CAD build for the part. Positions are in the model's coordinates, mm. Face numbers are marked on the shaded views. Round coordinates to 2 decimals unless told otherwise and drop trailing zeros. Loops run counter-clockwise (first coordinate to the right, second up) from the corner with the lowest first, then second, coordinate; pieces in that order, holes last. Notation, with made-up numbers: M 11.5,-25 L 27.5,-25 A19 cw 27.5,-17 Z; hole C -24,-36 d6. An arc over 180 degrees is marked long. Put each result on its own line as item: value. Start each with the question number.
from build123d import *
from build123d.topology import SkipClean

# Parameters (mm, degrees)
SCHIZZO1_R                   = 135
ESTRUSIONE_ESTRUSIONE2_DEPTH = 3
SCHIZZO4_R                   = 132
TAGLIO_ESTRUSIONE1_DEPTH     = 191.942399692
ESTRUSIONE_ESTRUSIONE3_DEPTH = 8
RIPETIZIONECIRCOLARE2_COUNT  = 4
ESTRUSIONE_ESTRUSIONE5_START = -3
ESTRUSIONE_ESTRUSIONE5_DEPTH = 3
RIPETIZIONECIRCOLARE4_COUNT  = 4
ESTRUSIONE_ESTRUSIONE6_START = 5
SCHIZZO9_R                   = 135
ESTRUSIONE_ESTRUSIONE6_DEPTH = 5
SCHIZZO10_R                  = 62.5
TAGLIO_ESTRUSIONE2_DEPTH     = 10
SCHIZZO11_R                  = 2.05
TAGLIO_ESTRUSIONE3_DEPTH     = 10


with BuildPart() as part:
    # Schizzo1 → Estrusione-Estrusione2 (new body)
    with BuildSketch(Plane.XY):
        Circle(SCHIZZO1_R)
    extrude(amount=ESTRUSIONE_ESTRUSIONE2_DEPTH)

    # Schizzo4 → Taglio-Estrusione1 (cut, through all)
    with BuildSketch(Plane.XY.offset(3)):
        Circle(SCHIZZO4_R)
    extrude(amount=-TAGLIO_ESTRUSIONE1_DEPTH, mode=Mode.SUBTRACT)

    # Schizzo5 → Estrusione-Estrusione3 (add)
    with SkipClean():  # the faces are left unmerged after this step: merging them gives an invalid solid
        with BuildSketch(Plane(origin=(0, 0, 0), x_dir=(-1, 0, 0), z_dir=(0, 0, -1))):
            with BuildLine():
                Line((-12.5, 134.420050588), (-12.5, 122.5))
                Line((-12.5, 122.5), (12.5, 122.5))
                Line((12.5, 122.5), (12.5, 134.420050588))
                ThreePointArc((12.5, 134.420050588), (0, 135), (-12.5, 134.420050588))
            make_face()
        estrusione_estrusione3 = extrude(amount=-ESTRUSIONE_ESTRUSIONE3_DEPTH)

    # RipetizioneCircolare2: Estrusione-Estrusione3 ×4 about axis
    with SkipClean():  # the faces are left unmerged after this step: merging them gives an invalid solid
        ripetizionecircolare2_axis = Axis((0, 0, 0), (0, 0, 1))
        for i in range(1, RIPETIZIONECIRCOLARE2_COUNT):
            add(estrusione_estrusione3.rotate(ripetizionecircolare2_axis, i * 360 / RIPETIZIONECIRCOLARE2_COUNT))

    # Schizzo8 → Estrusione-Estrusione5 (add)
    with SkipClean():  # the faces are left unmerged after this step: merging them gives an invalid solid
        with BuildSketch(Plane(origin=(0, 0, 0), x_dir=(-1, 0, 0), z_dir=(0, 0, -1)).offset(ESTRUSIONE_ESTRUSIONE5_START)):
            with BuildLine():
                Line((-12.5, 122.5), (12.5, 122.5))
                Line((12.5, 122.5), (32.648342939, 127.898732219))
                ThreePointArc((32.648342939, 127.898732219), (-42.175054348, 125.081032898), (-103.427881869, 82.016298697))
                Line((-103.427881869, 82.016298697), (-12.5, 122.5))
            make_face()
        estrusione_estrusione5 = extrude(amount=ESTRUSIONE_ESTRUSIONE5_DEPTH)

    # RipetizioneCircolare4: Estrusione-Estrusione5 ×4 about axis
    with SkipClean():  # the faces are left unmerged after this step: merging them gives an invalid solid
        ripetizionecircolare4_axis = Axis((0, 0, 0), (0, 0, 1))
        for i in range(1, RIPETIZIONECIRCOLARE4_COUNT):
            add(estrusione_estrusione5.rotate(ripetizionecircolare4_axis, i * 360 / RIPETIZIONECIRCOLARE4_COUNT))

    # Schizzo9 → Estrusione-Estrusione6 (add)
    with SkipClean():  # the faces are left unmerged after this step: merging them gives an invalid solid
        with BuildSketch(Plane(origin=(0, 0, 0), x_dir=(-1, 0, 0), z_dir=(0, 0, -1)).offset(ESTRUSIONE_ESTRUSIONE6_START)):
            Circle(SCHIZZO9_R)
        extrude(amount=-ESTRUSIONE_ESTRUSIONE6_DEPTH)

    # Schizzo10 → Taglio-Estrusione2 (cut)
    with SkipClean():  # the faces are left unmerged after this step: merging them gives an invalid solid
        with BuildSketch(Plane(origin=(0, 0, -5), x_dir=(-1, 0, 0), z_dir=(0, 0, -1))):
            Circle(SCHIZZO10_R)
        extrude(amount=-TAGLIO_ESTRUSIONE2_DEPTH, mode=Mode.SUBTRACT)

    # Schizzo11 → Taglio-Estrusione3 (cut)
    with SkipClean():  # the faces are left unmerged after this step: merging them gives an invalid solid
        with BuildSketch(Plane(origin=(0, 0, -5), x_dir=(-1, 0, 0), z_dir=(0, 0, -1))):
            with Locations((-91.168439698, -41.089117817)):
                Circle(SCHIZZO11_R)
            with Locations((-58.409625893, 81.168439698)):
                Circle(SCHIZZO11_R)
        extrude(amount=-TAGLIO_ESTRUSIONE3_DEPTH, mode=Mode.SUBTRACT)


solid = part.part
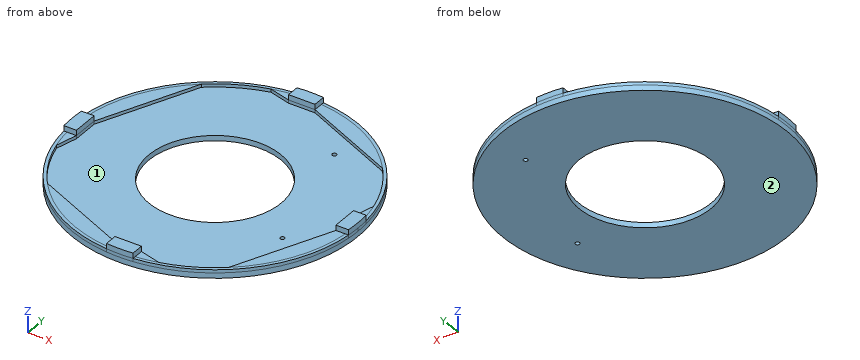
(1) Drill centre lines: line 1 along Y through (x, z) = (-2, 3); line 2 along Z through (x, y) = (31, -81.5); line 3 along Y through (x, z) = (0, -3.75). Where is each one in solid material? Low to high.
(2) Mould opens along Y. For the marked faces 1 and 2 say: +Y half, -Y half, draft (parallel to the pull), parting line (faces both ways), or undercut.
(3) Cut at A-A on z = 5.25. List the corners of the cut face in (x, y), and give its area (3 significant figures).
(4) Flat gauge pins, fed straight in: pin 1 Ø7 at (x, y) = (-21.5, 125) entering from +Z; pin 2 Ø10 at (x, y) = (55.5, -25.5) entering from -Z; pin 3 Ø1.5 at (x, z) = (-128.5, 5.5) entering from -Y; pin 4 Ø1.5 at (y, z) = (-129.5, 4.5) entering from -X. Where does each tip first touch, or does it go through?
(5) Cut at D-D on x = 67.5. List the corners of the cut face in (y, z), and give its area (3 significant figures).
(6) Cut at C-C on y = 24. List the corners of the cut face in (x, z).
(7) Cut at B-B on x = 0. List the corners of the cut face in (y, z), and give its area (3 significant figures).
Taken from the geometry:
1. line 1: -134.99 to -122.5, 122.5 to 134.99
1. line 2: -5 to 0
1. line 3: -135 to -62.5, 62.5 to 135
2. face 1: undercut
2. face 2: draft
3. outline: M -134.42,-12.5 L -122.5,-12.5 L -122.5,12.5 L -134.42,12.5 A135 ccw Z; M -12.5,-134.42 A135 ccw 12.5,-134.42 L 12.5,-122.5 L -12.5,-122.5 Z; M -12.5,122.5 L 12.5,122.5 L 12.5,134.42 A135 ccw -12.5,134.42 Z; M 122.5,-12.5 L 134.42,-12.5 A135 ccw 134.42,12.5 L 122.5,12.5 Z
3. area: 1,230 mm2
4. pin 1: z = 3
4. pin 2: z = -5
4. pin 3: y = -12.5
4. pin 4: x = -12.5
5. outline: M -116.91,-5 L 116.91,-5 L 116.91,3 L 98.01,3 L 98.01,0 L -113.44,0 L -113.44,3 L -116.91,3 Z
5. area: 1,240 mm2
6. outline: M -132.85,-5 L -57.71,-5 L -57.71,0 L -117.38,0 L -117.38,3 L -132.85,3 Z; M 57.71,-5 L 132.85,-5 L 132.85,3 L 125.58,3 L 125.58,0 L 57.71,0 Z
7. outline: M -135,-5 L -62.5,-5 L -62.5,0 L -122.5,0 L -122.5,8 L -135,8 Z; M 62.5,-5 L 135,-5 L 135,8 L 122.5,8 L 122.5,0 L 62.5,0 Z
7. area: 925 mm2
